Read the model definition and answer for the solid it produces. Units are mm, in the model's axes. A direction names the side the tool comes from. Give positions to 0.01 mm unless a question says otherwise; leave off trailing zeros. Write each loop counter-clockwise with the first axis right and the second up, starting at its lowest first coordinate (ties: lowest second). Pieces come first, ordered by that corner, then holes. Notation, with made-up numbers: (50, -21) -> (106, -21) arc R29 cw to (106, 3) -> close; hole circle Ø2 at (28.5, 25.5). An arc over 180 degrees is marked (long way). Write item = value, one per line.
from build123d import *

# Parameters (mm, degrees)
SKETCH_1_W          = 15
SKETCH_1_H          = 15
SKETCH_1_W_2        = 13
SKETCH_1_H_2        = 13
EXTRUDE_1_DEPTH     = 700
SKETCH_3_R          = 1.45
SKETCH_3_R_2        = 1.6
CUT_EXTRUDE_1_DEPTH = 701.200864038
SKETCH_4_R          = 1.45
SKETCH_4_R_2        = 1.6
CUT_EXTRUDE_2_DEPTH = 701.200864038


with BuildPart() as part:
    # 草图1 → 凸台-拉伸1 (new body)
    with BuildSketch(Plane(origin=(0, 0, 0), x_dir=(0, 0, -1), z_dir=(1, 0, 0))):
        Rectangle(SKETCH_1_W, SKETCH_1_H)
        Rectangle(SKETCH_1_W_2, SKETCH_1_H_2, mode=Mode.SUBTRACT)
    extrude(amount=EXTRUDE_1_DEPTH)

    # 草图3 → 切除-拉伸1 (cut, through all)
    with BuildSketch(Plane.XY.offset(7.5)):
        with Locations((595.5, 0)):
            Circle(SKETCH_3_R)
        with Locations((24, 0)):
            Circle(SKETCH_3_R)
        with Locations((14, 0)):
            Circle(SKETCH_3_R)
        with Locations((76.25, -0.621320344)):
            Circle(SKETCH_3_R_2)
        with Locations((66.25, -0.621320344)):
            Circle(SKETCH_3_R_2)
        with Locations((43.75, -0.621320344)):
            Circle(SKETCH_3_R_2)
        with Locations((33.75, -0.621320344)):
            Circle(SKETCH_3_R_2)
        with Locations((522.25, -0.621320344)):
            Circle(SKETCH_3_R_2)
        with Locations((512.25, -0.621320344)):
            Circle(SKETCH_3_R_2)
        with Locations((489.75, -0.621320344)):
            Circle(SKETCH_3_R_2)
        with Locations((479.75, -0.621320344)):
            Circle(SKETCH_3_R_2)
        with Locations((630.5, 0)):
            Circle(SKETCH_3_R)
        with Locations((547, 0)):
            Circle(SKETCH_3_R)
        with Locations((679, 0)):
            Circle(SKETCH_3_R)
    extrude(amount=-CUT_EXTRUDE_1_DEPTH, mode=Mode.SUBTRACT)

    # 草图4 → 切除-拉伸2 (cut, through all)
    with BuildSketch(Plane(origin=(0, 7.5, 0), x_dir=(1, 0, 0), z_dir=(0, 1, 0))):
        with Locations(Location((9, 0, 0), (0, 0, 270))):
            Circle(SKETCH_4_R)
        with Locations(Location((33.75, 0.621320344, 0), (0, 0, 270))):
            Circle(SKETCH_4_R_2)
        with Locations(Location((43.75, 0.621320344, 0), (0, 0, 270))):
            Circle(SKETCH_4_R_2)
        with Locations(Location((76.25, 0.621320344, 0), (0, 0, 270))):
            Circle(SKETCH_4_R_2)
        with Locations(Location((66.25, 0.621320344, 0), (0, 0, 270))):
            Circle(SKETCH_4_R_2)
        with Locations(Location((426, 0, 0), (0, 0, 270))):
            Circle(SKETCH_4_R)
        with Locations(Location((391, 0, 0), (0, 0, 270))):
            Circle(SKETCH_4_R)
        with Locations(Location((512.25, 0.621320344, 0), (0, 0, 270))):
            Circle(SKETCH_4_R_2)
        with Locations(Location((489.75, 0.621320344, 0), (0, 0, 270))):
            Circle(SKETCH_4_R_2)
        with Locations(Location((479.75, 0.621320344, 0), (0, 0, 270))):
            Circle(SKETCH_4_R_2)
        with Locations(Location((522.25, 0.621320344, 0), (0, 0, 270))):
            Circle(SKETCH_4_R_2)
        with Locations(Location((552, 0, 0), (0, 0, 270))):
            Circle(SKETCH_4_R)
        with Locations(Location((674, 0, 0), (0, 0, 270))):
            Circle(SKETCH_4_R)
        with Locations(Location((684, 0, 0), (0, 0, 270))):
            Circle(SKETCH_4_R)
        with Locations(Location((19, 0, 0), (0, 0, 270))):
            Circle(SKETCH_4_R)
        with Locations(Location((542, 0, 0), (0, 0, 270))):
            Circle(SKETCH_4_R)
    extrude(amount=-CUT_EXTRUDE_2_DEPTH, mode=Mode.SUBTRACT)


solid = part.part
(1) The part is cut by section A-A on x = 568. Determine the outline of the cut face in (y, z).
Checks:
outline = (-7.5, -7.5) -> (7.5, -7.5) -> (7.5, 7.5) -> (-7.5, 7.5) -> close; hole (-6.5, -6.5) -> (6.5, -6.5) -> (6.5, 6.5) -> (-6.5, 6.5) -> close
(2) Consider L1, parallel to Y at x = 559.5, z = -0.5; L2, parallel to Z at x = 552, y = -6.95. Determine where each line is inside the solid, lowest interval first.
Checks:
L1 = -7.5 to -6.5, 6.5 to 7.5
L2 = -7.5 to -1.45, 1.45 to 7.5
(3) For a pull along Y with two mould halves and no side action, classify faces 1 (the flat face through (700, 0, 7)), 2 (the flat face through (345, 7.5, 0)), 3 (the flat face through (345, 0, 6.5)) as released by +Y, released by -Y, zero draft, split by the parting line, or undercut.
Checks:
face_1 = zero draft
face_2 = released by +Y
face_3 = undercut
(4) A tool of negligible diameter and unlimited length cuts with its end or side. For faces 4 (the flat face through (0, 0, 7)), 5 (the flat face through (345, 6.5, 0)), from which of +Z, -Z, +X, -X, +Y, -Y can it reach the whole face along a straight path? Write none if from no direction.
Checks:
face_4 = +Z, -Z, -X, +Y, -Y
face_5 = +X, -X
